Autodesk Inventor part; units mm, degrees
ref_plane "Work Plane1" through (0, -20, 0) normal (0, 1, 0) x (-1, 0, 0)
ref_plane "Work Plane2" through (0, 16.5, 0) normal (0, -1, 0) x (1, 0, 0)
ref_plane "YZ Plane" through (0, 0, 0) normal (1, 0, 0) x (0, 1, 0)
sketch "Sketch2" plane through (0, 0, 0) normal (0, 0, 1) x (1, 0, 0)
  circle A0 centre (0, 0) radius 14
  circle A1 centre (0, 0) radius 12.5
  circle A2 centre (0, 0) radius 16.5
  circle A3 centre (0, 0) radius 15
  dimension "d0" = 28
  dimension "d1" = 25
  dimension "d2" = 33
  dimension "d3" = 30
extrude "Extrusion1" add sketch "Sketch2" against normal blind 10 contours A2 | A3
extrude "Extrusion2" add sketch "Sketch2" along normal blind 10 contours A0 | A3
ref_plane "Work Plane1" through (0, -20, 0) normal (0, 1, 0) x (-1, 0, 0)
sketch "Sketch3" plane through (0, -20, 0) normal (0, 1, 0) x (-1, 0, 0)
  line L0 (15, 10) -> (-15, 10)
  line L1 (-15, 0) -> (15, 0)
  line L2 (-26, 10) -> (-26, 0)
  line L3 (26, 10) -> (26, 0)
  line L4 (15, 0) -> (15, 10)
  line L5 (16.5, 0) -> (-16.5, 0)
  line L6 (-15, 0) -> (-16.5, 0)
  line L7 (-16.5, 0) -> (-16.5, 10)
  line L8 (-16.5, 10) -> (-15, 10)
  line L9 (16.5, 0) -> (16.5, 10)
  line L10 (16.5, 10) -> (15, 10)
  line L11 (-26, 0) -> (-16.5, 0)
  line L12 (-26, 10) -> (-16.5, 10)
  line L13 (16.5, 10) -> (26, 10)
  line L14 (-15, 0) -> (-15, 10)
  dimension "d9" = 11
  dimension "d10" = 11
  dimension "d11" = 10
  dimension "d36" = 33
extrude "Extrusion3" add sketch "Sketch3" along normal blind 20 contours L4 L1 L14 L0
extrude "Extrusion4" [suppressed]
extrude "Extrusion5" cut sketch "Sketch2" along normal through all contours A1
sketch "Sketch4" plane through (0, -10, 0) normal (0, 1, 0) x (1, 0, 0)
  line L0 (26, -10) -> (26, 0)
  line L1 (15, -10) -> (26, -10)
  line L2 (-26, -10) -> (-15, -10)
  line L3 (-26, 0) -> (-26, -10)
  point P0 (0, 0)
  point P1 (20.5, -4.5)
  point P2 (-21, -5)
  dimension "d18" = 5.5
  dimension "d19" = 5.5
  dimension "d20" = 5
  dimension "d21" = 5
hole "Hole1" [suppressed]
ref_plane "Work Plane2" through (0, 16.5, 0) normal (0, -1, 0) x (1, 0, 0)
sketch "Sketch5" plane through (0, 16.5, 0) normal (0, -1, 0) x (1, 0, 0)
  line L0 (-16.5, -10) -> (16.5, -10)
  line L1 (-3.75, -10) -> (3.75, -10)
  line L2 (3.75, -10) -> (3.75, -5.625)
  line L3 (3.75, -5.625) -> (-3.75, -5.625)
  line L4 (-3.75, -5.625) -> (-3.75, -10)
  arc A0 (3.75, -5.625) -> (-3.75, -5.625) centre (0, -5.625) ccw
  line L5 (15, 0) -> (-15, 0)
  circle A1 centre (0, -5.625) radius 2.125
  point P0 (0, 0)
  point P1 (0, 0)
  point P2 (-33, 0)
  point P3 (-33, 0)
  dimension "d29" = 3.75
extrude "Extrusion6" cut sketch "Sketch5" along normal blind 10
pattern_circular "Circular Pattern1" count 4 over 360 about axis through (0, 0, 0) along (0, 0, -1) of "Extrusion6"
sketch "Sketch6" plane through (0, -20, 0) normal (0, -1, 0) x (1, 0, 0)
  line L0 (15, 10) -> (15, 0)
  line L1 (-15, 0) -> (-15, 10)
  point P0 (0, 0)
  point P1 (10, 5)
  point P2 (-10, 5)
  point P3 (15, 5)
  point P4 (15, 5)
  dimension "d44" = 5
  dimension "d45" = 5
hole "Hole2" at (10, -20, 5) at (-10, -20, 5) direction (0, 1, 0) diameter 5.35 depth 10 tip angle 118
properties part number "Adafruit_1528_4699_ND_House_01"
Verification items for the finished model (mm, model axes). A direction names the side the tool comes from. Give positions to 0.01 mm unless a question says otherwise; leave off trailing zeros. Order: outer loops, then holes, each group sorted by start corner. A loop starts at its lowest first (then second) coordinate and runs counter-clockwise, first axis right, second up. Notation, with made-up numbers: M -8.75,-24.5 L 10.25,-24.5 A24 ccw 10.25,-11.5 Z; hole C 88,-38.5 d5. An arc over 180 degrees is marked long. Use one line per item in the form item = value. Start each with the question number.
Q1. Go/stop test with flat-tipped pins: pin 1 Ø3 at (y, z) = (-14.5, -7) entering from -X; pin 2 Ø4 at (y, z) = (6.5, 1) entering from -X; pin 3 Ø10 at (y, z) = (8, -3) entering from -X (3 decimals); pin 4 Ø11.5 at (x, y) = (1.5, 2.5) entering from +Z. Record where each tip stops, or that it passes through.
Q2. Mould release check, pull along X, two halves, no side actions. Record for faces 6 (the flat face through (0, -14, 10)), 7 (the conical face through (-10.41, -8.67, 4.79)), 8 (the cylindrical face through (15.24, -6.32, -4.93)): +X half, -X half, draft (parallel to the pull), parting line (faces both ways), or undercut.
Q3. Section check A-A (x = 0). Enter the section's corners in (y, z) (3 decimals).
Q4. Access from +Z, -Z, +X, -X, +Y, -Y to the whole of each face (thin tool, end or side, straight path). Record for faces 1 (the flat face through (-15, -10, 5)), 2 (the flat face through (-5.3, 11.5, 0)), 3 (the flat face through (-15, -3.75, -8)), 4 (the flat face through (-0.1, 15.3, 0)), 5 (the flat face through (3.75, 15, -8)).
Q5. Section check B-B (y = 10). Enter the section's corners in (x, z).
Q6. Scan lines: line 1 along Y through (x, z) = (0, 8); line 2 along Z through (x, y) = (10, -14) (3 decimals); line 3 along X through (y, z) = (-13.5, 5) (3 decimals). Record each from-to range of solid material in increasing order. Write a range as [from, to].
Q7. Section check C-C (z = 0.5). Enter the section's corners in (x, y), then the cut area to 3 significant figures.
Evaluation:
q1.pin_1 = -10.16
q1.pin_2 = -15.8
q1.pin_3 = -16.225
q1.pin_4 = through
q2.face_6 = draft
q2.face_7 = undercut
q2.face_8 = parting line
q3.outline = M -20,0 L -16.5,0 L -16.5,-1.875 L -14,-1.875 L -14,0 L -12.5,0 L -12.5,10 L -20,10 Z; M 12.5,0 L 14,0 L 14,-1.875 L 16.5,-1.875 L 16.5,0 L 15,0 L 15,10 L 12.5,10 Z
q4.face_1 = +Z, -X, +Y, -Y
q4.face_2 = -Z
q4.face_3 = -Z, +X, -X
q4.face_4 = +Z, +Y
q4.face_5 = -Z, +Y, -Y
q5.outline = M -13.12,-10 L -9.8,-10 L -9.8,0 L -7.5,0 L -7.5,10 L -11.18,10 L -11.18,0 L -13.12,0 Z; M 7.5,0 L 9.8,0 L 9.8,-10 L 13.12,-10 L 13.12,0 L 11.18,0 L 11.18,10 L 7.5,10 Z
q6.line_1 = [-20, -12.5], [12.5, 15]
q6.line_2 = [0, 2.325], [7.675, 10]
q6.line_3 = [-15, -12.675], [-7.325, 7.325], [12.675, 15]
q7.outline = M -15,-20 L 15,-20 L 15,0 A15 ccw -15,0 Z; hole C 0,0 d25
q7.area = 463 mm2
